from build123d import *

# Parameters (mm, degrees)
BASE_SKETCH_W                       = 55
BASE_SKETCH_H                       = 45
BASE_EXTRUDE_DEPTH                  = 6.5
RAISED_SECTION_SKETCH_W             = 37.5
RAISED_SECTION_SKETCH_H             = 22.5
RAISED_SECTION_EXTRUDE_DEPTH        = 3
MOSFET_MOUNTING_HOLES_D             = 1.6
MOUNTING_HOLES_D                    = 4.3053
MOUNTING_HOLES_CSINK_D              = 9.6944688
MOUNTING_HOLES_CSINK_ANGLE          = 82
CUT_PIN_RELIEF_DEPTH                = 54.136616377
CUT_PIN_RELIEF_DEPTH_BACK           = 54.136616377
PIN_SKETCH_W                        = 10
PIN_SKETCH_H                        = 12
PIN_SKETCH_W_2                      = 2
PIN_SKETCH_H_2                      = 10.5
LARGE_OUTSIDE_CORNER_FILLETS_R      = 8
SMALL_OUTSIDE_CORNER_FILLETS_R      = 2
SCREW_TERMINAL_CUTOUT_FILLETS_R     = 1
HEADER_PINS_CUTOUT_RELIEF_FILLETS_R = 1


with BuildPart() as part:
    # Base Sketch → Base Extrude (new body)
    with BuildSketch(Plane(origin=(0, 0, 0), x_dir=(1, 0, 0), z_dir=(0, 1, 0))):
        with Locations((0, 22.5)):
            Rectangle(BASE_SKETCH_W, BASE_SKETCH_H)
    extrude(amount=-BASE_EXTRUDE_DEPTH)

    # Raised Section Sketch → Raised Section Extrude (add)
    with BuildSketch(Plane(origin=(0, 0, 0), x_dir=(1, 0, 0), z_dir=(0, 1, 0))):
        with Locations((-8.75, 11.25)):
            Rectangle(RAISED_SECTION_SKETCH_W, RAISED_SECTION_SKETCH_H)
    extrude(amount=RAISED_SECTION_EXTRUDE_DEPTH)

    # Mosfet Mounting Holes (through all)
    with Locations(Plane(origin=(0, 3, 0), x_dir=(1, 0, 0), z_dir=(0, 1, 0))):
        with Locations((-23.5, 4), (-23.5, 17.5), (-8.5, 27.5), (-8.5, 41)):
            Hole(MOSFET_MOUNTING_HOLES_D / 2)

    # Mounting Holes (through all)
    with Locations(Plane(origin=(0, 0, 0), x_dir=(1, 0, 0), z_dir=(0, 1, 0))):
        with Locations((-20, 37.5), (20, 7.5)):
            CounterSinkHole(MOUNTING_HOLES_D / 2, MOUNTING_HOLES_CSINK_D / 2, counter_sink_angle=MOUNTING_HOLES_CSINK_ANGLE)

    # Pin Sketch → Cut Pin Relief (cut, two sides: drawn at the far end of the back side and taken through both)
    with BuildSketch(Plane(origin=(0, 0, 0), x_dir=(1, 0, 0), z_dir=(0, 1, 0)).offset(-CUT_PIN_RELIEF_DEPTH_BACK)):
        with Locations((2.5, 10.75)):
            Rectangle(PIN_SKETCH_W, PIN_SKETCH_H)
        with Locations((17.5, 34.25)):
            Rectangle(PIN_SKETCH_W, PIN_SKETCH_H)
        with Locations((-20.5, 10.75)):
            Rectangle(PIN_SKETCH_W_2, PIN_SKETCH_H_2)
        with Locations((-5.5, 34.25)):
            Rectangle(PIN_SKETCH_W_2, PIN_SKETCH_H_2)
    extrude(amount=CUT_PIN_RELIEF_DEPTH + CUT_PIN_RELIEF_DEPTH_BACK, mode=Mode.SUBTRACT)

    # Large Outside Corner Fillets
    large_outside_corner_fillets_edges = [part.edges().sort_by_distance(p)[0] for p in [
        (-27.5, -3.25, -45),
        (27.5, -3.25, 0),
    ]]
    fillet(large_outside_corner_fillets_edges, radius=LARGE_OUTSIDE_CORNER_FILLETS_R)

    # Small Outside Corner Fillets
    small_outside_corner_fillets_edges = [part.edges().sort_by_distance(p)[0] for p in [
        (-27.5, 1.5, -22.5),
        (10, 1.5, 0),
        (10, 1.5, -22.5),
        (27.5, -3.25, -45),
        (-27.5, -1.75, 0),
    ]]
    fillet(small_outside_corner_fillets_edges, radius=SMALL_OUTSIDE_CORNER_FILLETS_R)

    # Screw Terminal Cutout Fillets
    screw_terminal_cutout_fillets_edges = [part.edges().sort_by_distance(p)[0] for p in [
        (-2.5, -1.75, -4.75),
        (-2.5, -1.75, -16.75),
        (7.5, -1.75, -16.75),
        (7.5, -1.75, -4.75),
        (12.5, -3.25, -28.25),
        (12.5, -3.25, -40.25),
        (22.5, -3.25, -40.25),
        (22.5, -3.25, -28.25),
    ]]
    fillet(screw_terminal_cutout_fillets_edges, radius=SCREW_TERMINAL_CUTOUT_FILLETS_R)

    # Header Pins Cutout Relief Fillets
    header_pins_cutout_relief_fillets_edges = [part.edges().sort_by_distance(p)[0] for p in [
        (-4.5, -3.25, -29),
        (-6.5, -3.25, -29),
        (-6.5, -3.25, -39.5),
        (-4.5, -3.25, -39.5),
        (-19.5, -1.75, -16),
        (-21.5, -1.75, -16),
        (-21.5, -1.75, -5.5),
        (-19.5, -1.75, -5.5),
    ]]
    fillet(header_pins_cutout_relief_fillets_edges, radius=HEADER_PINS_CUTOUT_RELIEF_FILLETS_R - 0.0001)  # a hair under: the kernel refuses the full size


solid = part.part
For this review, take the finished solid that the model builds, in its own axes (mm). A direction names the side the tool comes from. Give positions to 0.01 mm unless a question says otherwise; leave off trailing zeros. Order: outer loops, then holes, each group sorted by start corner. A loop starts at its lowest first (then second) coordinate and runs counter-clockwise, first axis right, second up. Notation, with made-up numbers: M 57,76.25 L 115,76.25 A16 cw 115,93.25 Z; hole C 76.5,56.5 d8. An arc over 180 degrees is marked long. Answer in a Markdown table with one row per item. Add a question column.
(1) Consider section A-A on x = -8.5. State the section outline as (y, z) points.
(2) Consider section B-B on z = -17.5. State the section outline as (x, y) points.
(3) Mouldability with a two-part tool opening along X and no side actions: class faces 1 (the face through (-19.5, -2.95, -35.27)), 2 (the face through (3, -3, -45)), 3 (the face through (-27.5, -3, -19)) as +X half, -X half, draft (parallel to the pull), parting line (faces both ways), or undercut.
(4) For faces 4 (the face through (-9, 1, -22.5)), 5 (the face through (10, 1, -11)), 6 (the face through (2, -2, -4.75)), list the 3-axis set-ups (+Z, -Z, +X, -X, +Y, -Y) from which the entire face can be reached by the end or side of a thin tool; tool diameter is ignored.
(5) Wall thickness on probe 1 along X at (y, z) = (2, -9); probe 2 along Z at (x, y) = (-8.5, -2.25); probe 3 along X at (y, z) = (1, -17.5): over which ranges is each line inside the solid? List them lowest first. Write a range as [from, to].
(6) For pin 1 (2.5 mm diameter, centred on x = -8.5, z = -27.5, fed in from +Y), flat-tipped, find the tip position at first contact; note if it passes through.
(7) Consider section C-C on y = 1.5. Give the number of separate pieces and of enclosed holes in the cut face, and give its area (3 significant figures).
Evaluation:
| question | item | result |
|---|---|---|
| 1 | outline | M -6.5,-45 L 0,-45 L 0,-41.8 L -6.5,-41.8 Z; M -6.5,-40.2 L 0,-40.2 L 0,-28.3 L -6.5,-28.3 Z; M -6.5,-26.7 L 0,-26.7 L 0,-22.5 L 3,-22.5 L 3,0 L -6.5,0 Z |
| 2 | outline | M -27.5,-6.5 L -24.3,-6.5 L -24.3,3 L -27.5,3 Z; M -22.7,-6.5 L 27.5,-6.5 L 27.5,0 L 10,0 L 10,3 L -22.7,3 Z |
| 3 | face 1 | undercut |
| 3 | face 2 | draft |
| 3 | face 3 | -X half |
| 4 | face 4 | -Z, +X, -X, +Y |
| 4 | face 5 | +Z, -Z, +X, +Y |
| 4 | face 6 | +Y, -Y |
| 5 | probe 1 | x = [-27.5, -21.5], [-19.5, -2.5], [7.5, 10] |
| 5 | probe 2 | z = [-45, -41.8], [-40.2, -28.3], [-26.7, 0] |
| 5 | probe 3 | x = [-27.5, -24.3], [-22.7, 10] |
| 6 | pin 1 | stops at y = 0 |
| 7 | separate pieces | 1 |
| 7 | enclosed holes | 4 |
| 7 | area | 697 mm^2 |
